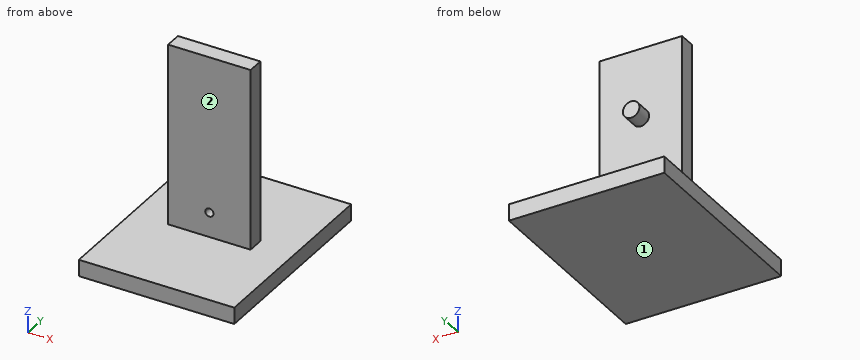
```python
from build123d import *

# Parameters (mm, degrees)
F0_W      = 127
F0_H      = 304.8
F1_DEPTH  = 25.4
F2_W      = 239.287932
F2_H      = 304.8
F2_W_2    = 127
F2_H_2    = 25.4
F3_DEPTH  = 25.4
F4_R      = 6.35
F5_DEPTH  = 167.098508
F6_R      = 12.7
F6_R_2    = 6.35
F7_DEPTH  = 32.258
F8_R      = 12.7
F9_DEPTH  = 50.8
F10_R     = 6.35
F11_DEPTH = 78.232


with BuildPart() as f1:
    # F0 (on Front) → F1 (new body)
    with BuildSketch(Plane.XZ):
        with Locations((3.56551, 32.600223)):
            Rectangle(F0_W, F0_H)
    extrude(amount=F1_DEPTH)

    # F2 (on face) → F3 (join)
    with BuildSketch(Plane(origin=(0, 0, -119.799777), x_dir=(1, 0, 0), z_dir=(0, 0, -1))):
        with Locations((3.56551, 10.702492)):
            Rectangle(F2_W, F2_H)
        with Locations((3.56551, 12.7)):
            Rectangle(F2_W_2, F2_H_2, mode=Mode.SUBTRACT)
    extrude(amount=-F3_DEPTH)

    # F4 (on face) → F5 (cut, through all)
    with BuildSketch(Plane.XZ.offset(25.4)):
        with Locations((3.56551, 77.050223)):
            Circle(F4_R)
    extrude(amount=-F5_DEPTH, mode=Mode.SUBTRACT)

    # F6 (on face) → F7 (cut)
    with BuildSketch(Plane(origin=(0, 0, 0), x_dir=(-1, 0, 0), z_dir=(0, 1, 0))):
        with Locations((-3.56551, 77.050223)):
            Circle(F6_R)
        with Locations((-3.56551, 77.050223)):
            Circle(F6_R_2, mode=Mode.SUBTRACT)
    extrude(amount=-F7_DEPTH, mode=Mode.SUBTRACT)

    # F8 (on face) → F9 (join)
    with BuildSketch(Plane.XZ.offset(25.4)):
        with Locations((3.56551, 77.050223)):
            Circle(F8_R)
    extrude(amount=-F9_DEPTH)

    # F10 (on face) → F11 (cut)
    with BuildSketch(Plane(origin=(0, 0, 0), x_dir=(-1, 0, 0), z_dir=(0, 1, 0))):
        with Locations((-3.56551, -56.299777)):
            Circle(F10_R)
    extrude(amount=-F11_DEPTH, mode=Mode.SUBTRACT)


solid = f1.part
```
Read the model definition and answer for the solid it produces. Units are mm, in the model's axes. Face numbers are marked on the shaded views. A direction names the side the tool comes from. Coordinates: 2 decimals unless noted, no trailing zeros. Write each loop counter-clockwise with the first axis right and the second up, starting at its lowest first coordinate (ties: lowest second). Pieces come first, ordered by that corner, then holes. Notation, with made-up numbers: (-19.5, 45) -> (-5.5, 45) arc R26 cw to (-5.5, 82) -> close; hole circle Ø11 at (47, 51.25). An arc over 180 degrees is marked (long way). Write item = value, one per line.
(1) Straight lines are drawn through the part: L1, parallel to Y at x = 60.5, z = -31; L2, parallel to Z at x = 71.5, y = -4.5; L3, parallel to X at y = -8, z = 146. For each, find the intervals that lie inside material, in ascending order. Write a range as from..to.
From the geometry:
L1 = -25.4..0
L2 = -119.8..-94.4
L3 = -59.93..67.07
(2) Which of the six approach directions +Z, -Z, +X, -X, +Y, -Y give full straight-line access (tool end or side, diameter ignored) to the marked faces 1 and 2?
From the geometry:
face_1 = -Z, +X, -X, +Y, -Y
face_2 = +Z, +X, -X, -Y
(3) Section C-C on y = -119.5 is taken. Write down the section's boundary in (x, z).
From the geometry:
outline = (-116.08, -119.8) -> (123.21, -119.8) -> (123.21, -94.4) -> (-116.08, -94.4) -> close
(4) Section D-D on z = -88 is taken. Write down the section's boundary in (x, y), plus the area to 3 significant figures.
From the geometry:
outline = (-59.93, -25.4) -> (67.07, -25.4) -> (67.07, 0) -> (-59.93, 0) -> close
area = 3,230 mm2
(5) Given pin 1 Ø7.5 at (y, z) = (-14.5, 67) entering from +X; pin 2 Ø7.5 at (x, z) = (9, 72.5) entering from +Y; pin 3 Ø8 at (x, z) = (64, -44.5) entering from +Y, each flat-ended and moving along its own axis, determine where each tip first touches the part or whether it passes through.
From the geometry:
pin_1 = 67.07
pin_2 = 25.4
pin_3 = 0
(6) Section B-B on x = 50 is taken. Write down the section's boundary in (y, z), plus the area to 3 significant figures.
From the geometry:
outline = (-163.1, -119.8) -> (141.7, -119.8) -> (141.7, -94.4) -> (0, -94.4) -> (0, 185) -> (-25.4, 185) -> (-25.4, -94.4) -> (-163.1, -94.4) -> close
area = 14,800 mm2
(7) Section A-A on x = 5.5 is taken. Write down the section's boundary in (y, z), plus the area to 3 significant figures.
From the geometry:
outline = (-163.1, -119.8) -> (141.7, -119.8) -> (141.7, -94.4) -> (0, -94.4) -> (0, -62.35) -> (-25.4, -62.35) -> (-25.4, -94.4) -> (-163.1, -94.4) -> close; (-25.4, -50.25) -> (0, -50.25) -> (0, 64.5) -> (25.4, 64.5) -> (25.4, 89.6) -> (0, 89.6) -> (0, 185) -> (-25.4, 185) -> close
area = 15,200 mm2
